The listing builds one solid part. Answer for the finished solid, in the listing's coordinates (mm). Coordinates: 2 decimals unless noted, no trailing zeros. Write each loop counter-clockwise with the first axis right and the second up, starting at its lowest first coordinate (ties: lowest second). Pieces come first, ordered by that corner, then holes.
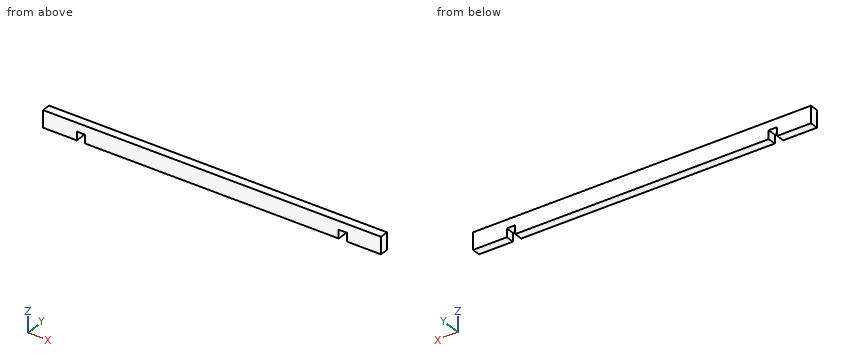
```python
from build123d import *

# Parameters (mm, degrees)
F0_W     = 50
F0_H     = 100
F1_DEPTH = 2000
F3_ANGLE = -90
F8_W     = 50
F8_H     = 50
F9_DEPTH = 50.001


with BuildPart() as f1:
    # F0 (on Right) → F1 (new body)
    with BuildSketch(Plane.YZ):
        Rectangle(F0_W, F0_H)
    extrude(amount=F1_DEPTH)

    # F8 (on face) → F9 (cut, through all)
    with BuildSketch(Plane.XZ.offset(25)):
        with Locations((225, -25)):
            Rectangle(F8_W, F8_H)
        with Locations((1775, -25)):
            Rectangle(F8_W, F8_H)
    extrude(amount=-F9_DEPTH, mode=Mode.SUBTRACT)


with BuildPart() as f2_1:
    # F2: copy of F1
    add(f1.part.moved(Location((0, 2000, 0))))


with BuildPart() as f3_1:
    # F3: copy of F1
    add(f1.part.rotate(Axis((0, -25, 0), (0, 0, 1)), F3_ANGLE))


with BuildPart() as f5_1:
    # F5: copy of F1
    add(f1.part)


solid = f1.part
```
(1) Find the intervals of material crossed by probe 1 along X at (y, z) = (-19, -6.5), in increasing order.
(2) Section A-A, the plane z = -16.5 is taken. Write down the section's boundary in (x, y), plus the area to 3 significant figures.
(3) Section B-B, the plane y = -8 is taken. Write down the section's boundary in (x, z).
(4) Each of these flat-tipped pins is pushed along its axis until it touches: pin 1 (15 mm diameter, centred on x = 1784, y = -4.5, fed in from -Z); pin 2 (6 mm diameter, centred on y = 16, z = -38.5, fed in from -X). Where does it stop, or does it pass through?
Solution:
1. probe 1: x = 0 to 200, 250 to 1750, 1800 to 2000
2. outline: (0, -25) - (200, -25) - (200, 25) - (0, 25) - close; (250, -25) - (1750, -25) - (1750, 25) - (250, 25) - close; (1800, -25) - (2000, -25) - (2000, 25) - (1800, 25) - close
2. area: 95,000 mm2
3. outline: (0, -50) - (200, -50) - (200, 0) - (250, 0) - (250, -50) - (1750, -50) - (1750, 0) - (1800, 0) - (1800, -50) - (2000, -50) - (2000, 50) - (0, 50) - close
4. pin 1: stops at z = 0
4. pin 2: stops at x = 0
